Could you check a few things on this model? Use its own coordinates, in mm. A direction names the side the tool comes from. Round coordinates to 2 decimals unless told otherwise and drop trailing zeros. Order: outer loops, then holes, each group sorted by start corner. A loop starts at its lowest first (then second) coordinate and runs counter-clockwise, first axis right, second up. Notation, with made-up numbers: M 55.25,-19.5 L 100.25,-19.5 A28 cw 100.25,2.5 Z; hole C 21.25,-5.5 d4. An arc over 180 degrees is marked long. Write each question's results on one line, items separated by ' | '. Start each with the question number.
1. For faces 1 (the flat face through (0, -2, 0)), 2 (the flat face through (-2.606, -6, 164)), 3 (the flat face through (-5, -3.195, 86)), 4 (the flat face through (-2.606, -6, 69)), 5 (the flat face through (0.394, -6, 155)), which set-ups out of +Z, -Z, +X, -X, +Y, -Y let a thin tool reach every point of the face, with its end or its side?
2. Please list where these lines run through material, in increasing order: L1, parallel to Y at x = -3, z = 55; L2, parallel to Z at x = 4.75, y = 1; L3, parallel to X at y = -3.5, z = 23.
3. Suppose I cut it at C-C on y = 2.75. Write out the boundary of the cut face in (x, z).
4. I'm going to push flat-ended pins straight in: pin 1 (4 mm diameter, centred on y = -7, z = 103, fed in from +X); pin 2 (5 mm diameter, centred on x = 3.5, y = 2.5, fed in from -Z); pin 3 (2.5 mm diameter, centred on x = -5, z = 114, fed in from +Y); pin 4 (5.5 mm diameter, centred on y = -6, z = 162.5, fed in from +X). Where does each tip first touch, or does it pass through?
5. Suppose I cut it at A-A on x = -4.5. Write out the boundary of the cut face in (y, z).
6. Suppose I cut it at B-B on z = 125.5. Write out the boundary of the cut face in (x, y).
from build123d import *

# Parameters (mm, degrees)
SKETCH007_W  = 15
SKETCH007_H  = 13
PAD007_DEPTH = 2
SKETCH008_W  = 5
SKETCH008_H  = 5
PAD008_DEPTH = 153
SKETCH009_W  = 5
SKETCH009_H  = 33.74
PAD009_DEPTH = 3


with BuildPart() as part:
    # Sketch007 → Pad007 (new body)
    with BuildSketch(Plane.XY):
        with Locations((-0.106383, -1.694786)):
            Rectangle(SKETCH007_W, SKETCH007_H)
    extrude(amount=PAD007_DEPTH)

    # Sketch008 (on Face6 of Pad007) → Pad008 (join)
    with BuildSketch(Plane.XY.offset(2)):
        with Locations((-5.106383, -5.694786)):
            Rectangle(SKETCH008_W, SKETCH008_H)
    extrude(amount=PAD008_DEPTH)

    # Sketch009 (on Face5 of Pad008) → Pad009 (join)
    with BuildSketch(Plane.YZ.offset(-2.606383)):
        with Locations((-5.694786, 155)):
            Rectangle(SKETCH009_W, SKETCH009_H)
    extrude(amount=PAD009_DEPTH)


solid = part.part
Filled sheet:
1) face 1: -Z, +X, -X, +Y, -Y | face 2: +Z, -X, +Y, -Y | face 3: +Z, +X, -X, +Y | face 4: +X, +Y, -Y | face 5: +Z, +X, +Y, -Y
2) L1: y = -8.19 to -3.19 | L2: z = 0 to 2 | L3: x = -7.61 to -2.61
3) outline: M -7.61,0 L 7.39,0 L 7.39,2 L -7.61,2 Z
4) pin 1: stops at x = -2.61 | pin 2: stops at z = 0 | pin 3: stops at y = -3.19 | pin 4: stops at x = 0.39
5) outline: M -8.19,0 L 4.81,0 L 4.81,2 L -3.19,2 L -3.19,155 L -8.19,155 Z
6) outline: M -7.61,-8.19 L -2.61,-8.19 L -2.61,-3.19 L -7.61,-3.19 Z
